Part print with two shaded views. Sizes in mm from the minimum x, y, z corner. Give positions to 0.01 mm unless a question says otherwise; leave off trailing zeros. Order: outer loops, then holes, each group sorted by start corner. A loop starts at its lowest first (then second) coordinate and runs counter-clockwise, first axis right, second up. Notation, with made-up numbers: (2, 59.5) - (54, 59.5) arc R17 cw to (54, 74.5) - close; hole circle Ø8 at (-25.5, -1). An arc over 180 degrees is marked (long way). Return JSON: item names as keys, results as strings. Group by question number.
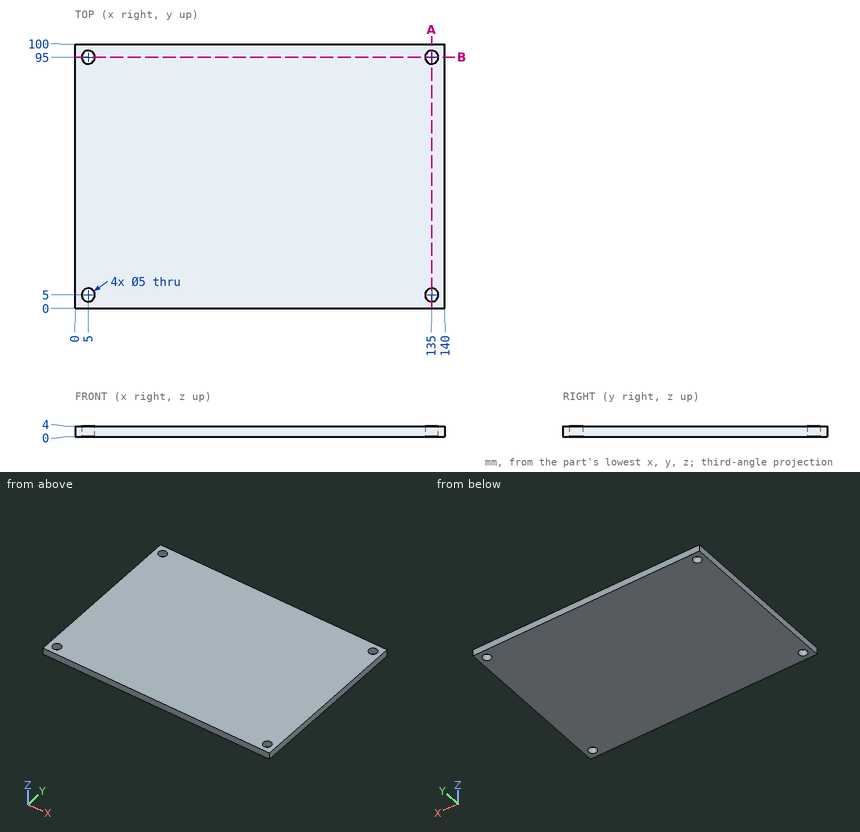
(1) Slice it at B-B (y = 95). Give the cut face in (x, z).
(2) Drop flat-ended pins along their axis: pin 1 Ø6.5 at (x, y) = (135, 5) entering from -Z; pin 2 Ø4.5 at (x, y) = (5, 5) entering from +Z. Give the stop position or say it passes through.
(3) Drill centre lines: L1, parallel to X at y = 95, z = 2.8; L2, parallel to Y at x = 135, z = 2.6; L3, parallel to X at y = 5.5, z = 0.7. Where is each one in solid material? Low to high.
(4) Slice it at A-A (x = 135). Give the cut face in (y, z).
Result set:
{
 "1": {"outline": "(0, 0) - (2.5, 0) - (2.5, 4) - (0, 4) - close; (7.5, 0) - (132.5, 0) - (132.5, 4) - (7.5, 4) - close; (137.5, 0) - (140, 0) - (140, 4) - (137.5, 4) - close"},
 "2": {"pin 1": "stops at z = 0", "pin 2": "passes through"},
 "3": {"L1": "x = 0 to 2.5, 7.5 to 132.5, 137.5 to 140", "L2": "y = 0 to 2.5, 7.5 to 92.5, 97.5 to 100", "L3": "x = 0 to 2.55, 7.45 to 132.55, 137.45 to 140"},
 "4": {"outline": "(0, 0) - (2.5, 0) - (2.5, 4) - (0, 4) - close; (7.5, 0) - (92.5, 0) - (92.5, 4) - (7.5, 4) - close; (97.5, 0) - (100, 0) - (100, 4) - (97.5, 4) - close"}
}
